```python
from build123d import *

# Parameters (mm, degrees)
EXTRUDE1_DEPTH                               = 8.6995
EXTRUDE1_DEPTH_BACK                          = 8.6995
SKETCH1_W                                    = 31.75
SKETCH1_H                                    = 31.75
F_056_250_NOSE_CHAMFER_R                     = 0.4
SKETCH13_R                                   = 22.450640303
SKETCH13_R_2                                 = 19.82
F_075_250_TUBE_EDGE_ROUNDOVER_DEPTH          = 29.403458434
F_075_250_PORT_BOSS_DEPTH                    = 17.399
F_075_PORT_10_32_AT_2_COUNT                  = 2
F_075_PORT_10_32_AT_2_PITCH                  = 7.747
F_075_250_SWITCH_GROOVE_DEPTH                = 30.321784581
F_075_106_SWITCH_GROOVE_CIRC_PATTERN_COUNT   = 3
F_075_106_SWITCH_GROOVE_CIRC_PATTERN_ANGLE   = 180
SKETCH19_W                                   = 0.15
SKETCH19_H                                   = 7
F_075_250_THIN_SIDE_CUTS_DEPTH               = 30.321784581
SKETCH20_R                                   = 1.95
F_075_250_MOUNT_THRU_HOLE_DEPTH              = 30.321784581
F_075_250_MOUNT_THRU_HOLE_CIRC_PATTERN_COUNT = 4
SKETCH21_R                                   = 3.175
F_075_250_B_MOUNT_CBORE_ROD_END_DEPTH        = 3.81
F_056_250_START                              = -4.0875
SKETCH22_R                                   = 9.525
F_056_250_STROKE_CHAMBER_DEPTH               = 8.175
SKETCH23_R                                   = 3.937
F_056_250_ROD_THRU_BORE_DEPTH                = 26.153988754
F_056_250_COLLAR_CHAMFER_SIZE                = 0.2


with BuildPart() as part:
    # Sketch1 → Extrude1 (new, two sides: drawn at the far end of the back side and taken through both)
    with BuildSketch(Plane.XY.offset(-EXTRUDE1_DEPTH_BACK)):
        Rectangle(SKETCH1_W, SKETCH1_H)
    extrude(amount=EXTRUDE1_DEPTH + EXTRUDE1_DEPTH_BACK)

    # Sketch33 → 056-250 Front Recess (revolve, cut)
    with BuildSketch(Plane(origin=(0, 0, 0), x_dir=(0, 0, -1), z_dir=(1, 0, 0)), mode=Mode.PRIVATE) as f_056_250_front_recess_sk:
        Polygon((-8.6995, 10), (-7.5495, 10), (-7.5495, 10.5), (-6.5745, 10.5), (-6.5745, 6), (-8.6995, 6), align=None)
    revolve(f_056_250_front_recess_sk.sketch.rotate(Axis((0, 0, 61.220394237), (0, 0, -1)), 90), axis=Axis((0, 0, 61.220394237), (0, 0, -1)), mode=Mode.SUBTRACT)

    # 056-250 Nose Chamfer
    f_056_250_nose_chamfer_edges = [part.edges().sort_by_distance(p)[0] for p in [
        (-6, 0, 6.5745),
    ]]
    fillet(f_056_250_nose_chamfer_edges, radius=F_056_250_NOSE_CHAMFER_R)

    # Sketch13 → 075-250 Tube Edge Roundover (cut, through all)
    with BuildSketch(Plane.XY.offset(8.6995)):
        Circle(SKETCH13_R)
        Circle(SKETCH13_R_2, mode=Mode.SUBTRACT)
    extrude(amount=-F_075_250_TUBE_EDGE_ROUNDOVER_DEPTH, mode=Mode.SUBTRACT)

    # Sketch14 → 075-250 Port Boss (add)
    with BuildSketch(Plane.XY.offset(8.6995)):
        Polygon((-4.75, 17.465), (4.75, 17.465), (4.889106975, 15.875), (-4.889106975, 15.875), align=None)
    extrude(amount=-F_075_250_PORT_BOSS_DEPTH)

    # Sketch35 → 075  Port #10-32 (revolve, cut)
    with BuildSketch(Plane(origin=(0, 17.465, 3.8735), x_dir=(0, 0, 1), z_dir=(1, 0, 0))):
        Polygon((0, 0), (0, 7.590757848), (2.0193, 6.37744), (2.0193, 4), (2.413, 4), (2.413, 0.934287129), (2.7999944, 0), align=None)
    f_075_port_10_32 = revolve(axis=Axis((0, 23.815, 3.8735), (0, -1, 0)), mode=Mode.SUBTRACT)

    # 075  Port #10-32 at 2: 075  Port #10-32 ×2
    with Locations(*[(0, 0, -i * F_075_PORT_10_32_AT_2_PITCH) for i in range(1, F_075_PORT_10_32_AT_2_COUNT)]):
        add(f_075_port_10_32, mode=Mode.SUBTRACT)

    # Sketch15 → 075-250 Switch Groove (cut, through all)
    with BuildSketch(Plane.XY.offset(8.6995)):
        with BuildLine():
            Line((-15.875, 6.5), (-14.235376786, 6.5))
            ThreePointArc((-14.235376786, 6.5), (-10.85, 5), (-14.235376786, 3.5))
            Line((-14.235376786, 3.5), (-15.875, 3.5))
            Line((-15.875, 3.5), (-15.875, 6.5))
        make_face()
        with BuildLine():
            Line((-15.875, -6.5), (-15.875, -3.5))
            Line((-15.875, -3.5), (-14.235376786, -3.5))
            ThreePointArc((-14.235376786, -3.5), (-10.85, -5), (-14.235376786, -6.5))
            Line((-14.235376786, -6.5), (-15.875, -6.5))
        make_face()
    f_075_250_switch_groove = extrude(amount=-F_075_250_SWITCH_GROOVE_DEPTH, mode=Mode.SUBTRACT)

    # 075-106 Switch Groove Circ Pattern: 075-250 Switch Groove ×3 about axis
    f_075_106_switch_groove_circ_pattern_axis = Axis((0, 0, 0), (0, 0, 1))
    for i in range(1, F_075_106_SWITCH_GROOVE_CIRC_PATTERN_COUNT):
        add(f_075_250_switch_groove.rotate(f_075_106_switch_groove_circ_pattern_axis, i * F_075_106_SWITCH_GROOVE_CIRC_PATTERN_ANGLE / (F_075_106_SWITCH_GROOVE_CIRC_PATTERN_COUNT - 1)), mode=Mode.SUBTRACT)

    # Sketch19 → 075-250 Thin Side Cuts (cut, through all)
    with BuildSketch(Plane.XY.offset(8.6995)):
        with Locations((15.8, 0)):
            Rectangle(SKETCH19_W, SKETCH19_H)
        with Locations((-15.8, 0)):
            Rectangle(SKETCH19_W, SKETCH19_H)
    extrude(amount=-F_075_250_THIN_SIDE_CUTS_DEPTH, mode=Mode.SUBTRACT)

    # Sketch20 → 075-250 Mount Thru Hole (cut, through all)
    with BuildSketch(Plane.XY.offset(8.6995)):
        with Locations((10.945, 10.945)):
            Circle(SKETCH20_R)
    f_075_250_mount_thru_hole = extrude(amount=-F_075_250_MOUNT_THRU_HOLE_DEPTH, mode=Mode.SUBTRACT)

    # 075-250 Mount Thru Hole Circ Pattern: 075-250 Mount Thru Hole ×4 about axis
    f_075_250_mount_thru_hole_circ_pattern_axis = Axis((0, 0, 0), (0, 0, 1))
    for i in range(1, F_075_250_MOUNT_THRU_HOLE_CIRC_PATTERN_COUNT):
        add(f_075_250_mount_thru_hole.rotate(f_075_250_mount_thru_hole_circ_pattern_axis, i * 360 / F_075_250_MOUNT_THRU_HOLE_CIRC_PATTERN_COUNT), mode=Mode.SUBTRACT)

    # Sketch21 → 075-250 B Mount CBore Rod End (cut)
    with BuildSketch(Plane.XY.offset(8.6995)):
        with Locations((-10.945, 10.945)):
            Circle(SKETCH21_R)
        with Locations((-10.945, -10.945)):
            Circle(SKETCH21_R)
        with Locations((10.945, 10.945)):
            Circle(SKETCH21_R)
        with Locations((10.945, -10.945)):
            Circle(SKETCH21_R)
    f_075_250_b_mount_cbore_rod_end = extrude(amount=-F_075_250_B_MOUNT_CBORE_ROD_END_DEPTH, mode=Mode.SUBTRACT)

    # 075-250 B Mount CBore Non-Rod End: 075-250 B Mount CBore Rod End across plane
    add(f_075_250_b_mount_cbore_rod_end.mirror(Plane.XY), mode=Mode.SUBTRACT)

    # Sketch22 → 056-250 Stroke Chamber (cut)
    with BuildSketch(Plane.XY.offset(F_056_250_START)):
        Circle(SKETCH22_R)
    extrude(amount=F_056_250_STROKE_CHAMBER_DEPTH, mode=Mode.SUBTRACT)

    # Sketch23 → 056-250 Rod Thru Bore (cut, through all)
    with BuildSketch(Plane.XY):
        with Locations(Location((0, 0, 0), (0, 0, 180))):
            Circle(SKETCH23_R)
    extrude(amount=F_056_250_ROD_THRU_BORE_DEPTH, mode=Mode.SUBTRACT)

    # 056-250 Collar Chamfer
    f_056_250_collar_chamfer_edges = [part.edges().sort_by_distance(p)[0] for p in [
        (-10, 0, 8.6995),
        (-6, 0, 8.6995),
        (3.937, 0, 8.6995),
    ]]
    chamfer(f_056_250_collar_chamfer_edges, length=F_056_250_COLLAR_CHAMFER_SIZE)


solid = part.part
```
The listing builds one solid part. Answer for the finished solid, in the listing's coordinates (mm). A direction names the side the tool comes from. Give positions to 0.01 mm unless a question says otherwise; leave off trailing zeros. Answer in a Markdown table with one row per item. Add a question column.
Q1. Find the intervals of material crossed by line 1 along Z through (x, y) = (1, -6.5); line 2 along X through (y, z) = (11, -4) (3 decimals); line 3 along Y through (x, z) = (10, 1.5) (3 decimals), in increasing order. Write a range as [from, to].
Q2. Which of the six approach directions +Z, -Z, +X, -X, +Y, -Y give full straight-line access (tool end or side, diameter ignored) to faces 1 (the cylindrical face through (-11.358, -7.797, 6.821)), 2 (the flat face through (15, -3.5, 0)), 3 (the flat face through (-15, 3.5, 0)), 4 (the flat face through (-8, 15.875, 0))?
Q3. The part is cut by section A-A (z = -3). Give the number of separate pieces and of enclosed holes in the cut face, then the cut area to 3 significant figures.
Q4. Given P1, Ø5, axis at x = 10.945, y = -10.945, coming from the +Z side; P2, Ø1.9, axis at x = 11.5, y = 12, coming from the -Z side; P3, Ø1.3, axis at y = -15, z = 2, coming from the -X side, each flat-ended and moving along its own axis, determine where each tip first touches the part or whether it passes through.
Q5. For a pull along Z with two mould halves and no side action, classify faces 5 (the flat face through (-10, -9, -4.89)), 6 (the cylindrical face through (-0.72, 15.02, -1.57)), 7 (the cylindrical face through (8.605, -8.799, 6.821)) as released by +Z, released by -Z, zero draft, split by the parting line, or undercut.
Determined:
| question | item | result |
|---|---|---|
| 1 | line 1 | z = [-8.7, -4.09], [4.09, 6.57] |
| 1 | line 2 | x = [-15.875, -12.894], [-8.996, -1.869], [1.869, 8.996], [12.894, 15.875] |
| 1 | line 3 | y = [-15.875, -12.651], [-9.239, 9.239], [12.651, 15.875] |
| 2 | face 1 | +Z |
| 2 | face 2 | +Z, -Z, +X |
| 2 | face 3 | +Z, -Z, -X |
| 2 | face 4 | +Z, -Z, -X, +Y |
| 3 | separate pieces | 1 |
| 3 | enclosed holes | 5 |
| 3 | area | 532 mm² |
| 4 | P1 | stops at z = 4.89 |
| 4 | P2 | stops at z = -4.89 |
| 4 | P3 | stops at x = -13.67 |
| 5 | face 5 | released by -Z |
| 5 | face 6 | undercut |
| 5 | face 7 | zero draft |
